Check sheet for the drawn part. Datum: minimum x, y, z corner. Units: mm. A direction names the side the tool comes from. Round coordinates to 2 decimals unless told otherwise and drop trailing zeros. Write each loop counter-clockwise with the first axis right and the second up, starting at its lowest first coordinate (ties: lowest second). Pieces come first, ordered by that corner, then holes.
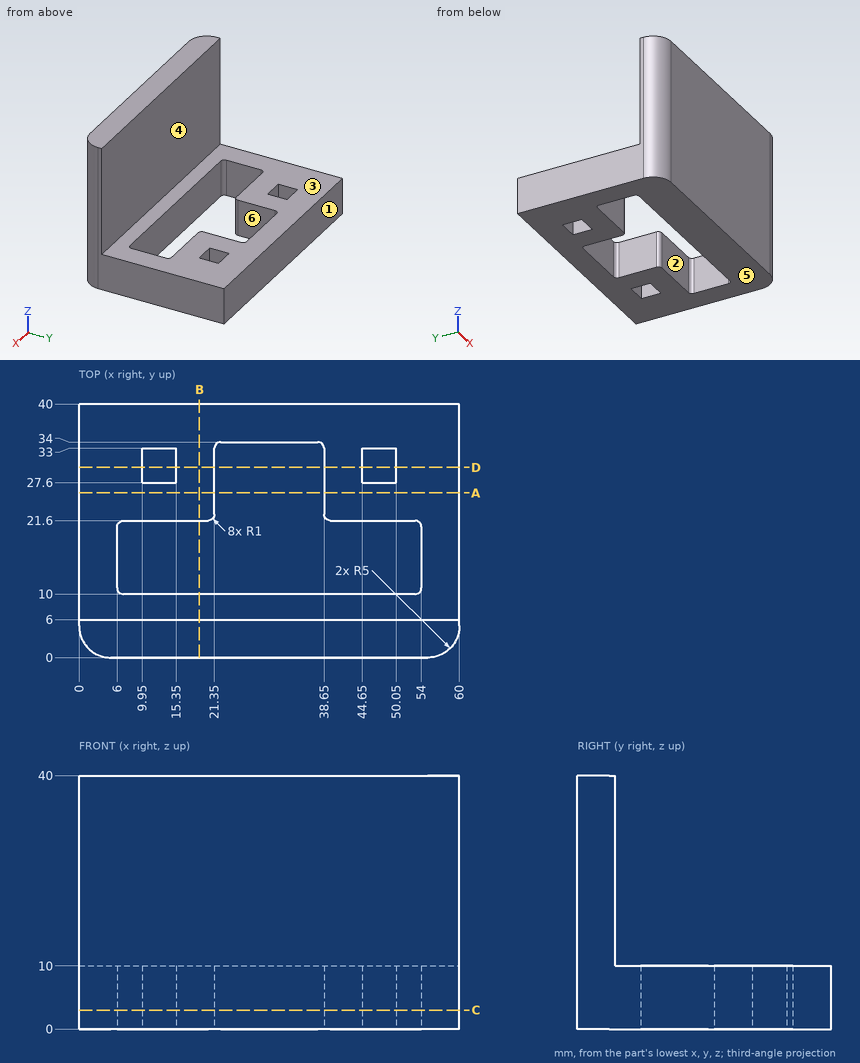
1. Scan lines: line 1 along X through (y, z) = (30, 2); line 2 along Y through (x, z) = (32, 6); line 3 along Y through (x, z) = (9.5, 20). Record each from-to range of solid material in increasing order.
2. Release check for a two-part mould opening along Y. For the marked faces 4, 5 and 6 record: released by +Y, released by -Y, zero draft, split by the parting line, or undercut.
3. Set-up check for the marked faces 1, 2 and 3: record each of +Z, -Z, +X, -X, +Y, -Y from which the full face is reachable in a straight line by a thin tool's end or side.
4. Go/stop test with flat-tipped pins: pin 1 (6 mm diameter, centred on x = 18, y = 10.5, fed in from +Z); pin 2 (9 mm diameter, centred on x = 33.5, z = 22, fed in from +Y). Record where each tip stops, or that it passes through.
5. Sectioned sample at A-A, the plane y = 26. Enter the section's corners in (x, z), plus the area to 3 significant figures.
6. Sectioned sample at B-B, the plane x = 19. Enter the section's corners in (y, z).
7. Sectioned sample at D-D, the plane y = 30. Enter the section's corners in (x, z).
8. Sectioned sample at C-C, the plane z = 3. Give the number of separate pieces and of enclosed holes in the cut face, plus the area to 3 significant figures.
Computed values:
1. line 1: x = 0 to 9.95, 15.35 to 21.35, 38.65 to 44.65, 50.05 to 60
1. line 2: y = 0 to 10, 34 to 40
1. line 3: y = 0 to 6
2. face 4: released by +Y
2. face 5: zero draft
2. face 6: undercut
3. face 1: +Z, -Z, +X, -X, +Y
3. face 2: +Z, -Z
3. face 3: +Z, +X, -X, +Y
4. pin 1: stops at z = 10
4. pin 2: stops at y = 6
5. outline: (0, 0) - (21.35, 0) - (21.35, 10) - (0, 10) - close; (38.65, 0) - (60, 0) - (60, 10) - (38.65, 10) - close
5. area: 427 mm2
6. outline: (0, 0) - (10, 0) - (10, 10) - (6, 10) - (6, 40) - (0, 40) - close; (21.6, 0) - (40, 0) - (40, 10) - (21.6, 10) - close
7. outline: (0, 0) - (9.95, 0) - (9.95, 10) - (0, 10) - close; (15.35, 0) - (21.35, 0) - (21.35, 10) - (15.35, 10) - close; (38.65, 0) - (44.65, 0) - (44.65, 10) - (38.65, 10) - close; (50.05, 0) - (60, 0) - (60, 10) - (50.05, 10) - close
8. separate pieces: 1
8. enclosed holes: 3
8. area: 1,560 mm2
